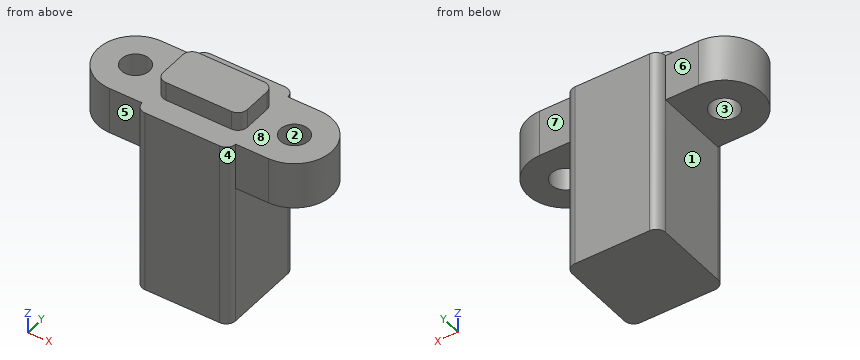
from build123d import *

# Parameters (mm, degrees)
SKETCH2_R           = 1.5
BOSS_EXTRUDE1_DEPTH = 5
BOSS_EXTRUDE2_DEPTH = 2
BOSS_EXTRUDE3_START = -15
SKETCH2_3_W         = 10
SKETCH2_3_H         = 4
BOSS_EXTRUDE3_DEPTH = 15


with BuildPart() as part:
    # Sketch2 → Boss-Extrude1 (new body)
    # profile 1 of 2: a face of its own
    with BuildSketch(Plane.XY):
        with BuildLine():
            Line((0, -4), (-17, -4))
            ThreePointArc((-17, -4), (-21, 0), (-17, 4))
            Line((-17, 4), (0, 4))
            ThreePointArc((0, 4), (4, 0), (0, -4))
        make_face()
        with Locations((-17, 0)):
            Circle(SKETCH2_R, mode=Mode.SUBTRACT)
        Circle(SKETCH2_R, mode=Mode.SUBTRACT)
    # profile 2 of 2: a face of its own
    with BuildSketch(Plane.XY):
        with BuildLine():
            Line((-12.5, 5), (-4.5, 5))
            ThreePointArc((-4.5, 5), (-3.792893219, 4.707106781), (-3.5, 4))
            Line((-3.5, 4), (-3.5, -4))
            ThreePointArc((-3.5, -4), (-3.792893219, -4.707106781), (-4.5, -5))
            Line((-4.5, -5), (-12.5, -5))
            ThreePointArc((-12.5, -5), (-13.207106781, -4.707106781), (-13.5, -4))
            Line((-13.5, -4), (-13.5, 4))
            ThreePointArc((-13.5, 4), (-13.207106781, 4.707106781), (-12.5, 5))
        make_face()
    extrude(amount=BOSS_EXTRUDE1_DEPTH)

    # Sketch3 → Boss-Extrude2 (add)
    with BuildSketch(Plane.XY.offset(5)):
        with BuildLine():
            Line((-12, -2.5), (-5, -2.5))
            ThreePointArc((-5, -2.5), (-4.292893219, -2.207106781), (-4, -1.5))
            Line((-4, -1.5), (-4, 1.5))
            ThreePointArc((-4, 1.5), (-4.292893219, 2.207106781), (-5, 2.5))
            Line((-5, 2.5), (-12, 2.5))
            ThreePointArc((-12, 2.5), (-12.707106781, 2.207106781), (-13, 1.5))
            Line((-13, 1.5), (-13, -1.5))
            ThreePointArc((-13, -1.5), (-12.707106781, -2.207106781), (-12, -2.5))
        make_face()
    extrude(amount=BOSS_EXTRUDE2_DEPTH)

    # Sketch2_3 → Boss-Extrude3 (add)
    with BuildSketch(Plane.XY.offset(BOSS_EXTRUDE3_START)):
        with BuildLine():
            Line((-13.5, 4), (-3.5, 4))
            ThreePointArc((-3.5, 4), (-3.792893219, 4.707106781), (-4.5, 5))
            Line((-4.5, 5), (-12.5, 5))
            ThreePointArc((-12.5, 5), (-13.207106781, 4.707106781), (-13.5, 4))
        make_face()
        with Locations((-8.5, 2)):
            Rectangle(SKETCH2_3_W, SKETCH2_3_H)
        with Locations((-8.5, -2)):
            Rectangle(SKETCH2_3_W, SKETCH2_3_H)
        with BuildLine():
            ThreePointArc((-4.5, -5), (-3.792893219, -4.707106781), (-3.5, -4))
            Line((-3.5, -4), (-13.5, -4))
            ThreePointArc((-13.5, -4), (-13.207106781, -4.707106781), (-12.5, -5))
            Line((-12.5, -5), (-4.5, -5))
        make_face()
    extrude(amount=BOSS_EXTRUDE3_DEPTH)


solid = part.part
Design review of the part built by this model. Coordinates are the model's own, in mm. Face numbers are marked on the shaded views. A direction names the side the tool comes from. Round coordinates to 2 decimals unless told otherwise and drop trailing zeros. Loops run counter-clockwise (first coordinate to the right, second up) from the corner with the lowest first, then second, coordinate; pieces in that order, holes last. Notation, with made-up numbers: (16.25, -16.5) - (66.25, -16.5) arc R31 cw to (66.25, 9.5) - close; hole circle Ø3 at (70.25, 5). An arc over 180 degrees is marked (long way). One line per question, with ' | ' between items.
1. We need section D-D, the plane z = -11. State the section outline as (x, y) points, and give its area (3 significant figures).
Results are:
outline: (-13.5, -4) arc R1 ccw to (-12.5, -5) - (-4.5, -5) arc R1 ccw to (-3.5, -4) - (-3.5, 4) arc R1 ccw to (-4.5, 5) - (-12.5, 5) arc R1 ccw to (-13.5, 4) - close | area: 99.1 mm²
2. For the marked faces 5, 6, 7 and 8, list the 3-axis set-ups (+Z, -Z, +X, -X, +Y, -Y) from which the entire face can be reached by the end or side of a thin tool; tool diameter is ignored.
Results are:
face 5: +Z, -Z, -X, -Y | face 6: +Z, -Z, -X, +Y | face 7: +Z, -Z, +X, +Y | face 8: +Z
3. Clearance check with flat-ended pins moving along their axes: P1, Ø1.6, axis at x = -9, z = 6.5, coming from the -Y side; P2, Ø4, axis at y = 2, z = -8, coming from the -X side; P3, Ø4, axis at y = 1, z = -10, coming from the +X side; P4, Ø6, axis at y = -1, z = 3.5, coming from the +X side. State where each tip first meets the part, or that it passes through.
Results are:
P1: stops at y = -2.5 | P2: stops at x = -13.5 | P3: stops at x = -3.5 | P4: stops at x = 4
4. Draft analysis for pull direction Y (two halves, no side actions). For the marked faces 1, 2, 3 and 4, state which applies: released by +Y, released by -Y, zero draft, split by the parting line, or undercut.
Results are:
face 1: zero draft | face 2: undercut | face 3: undercut | face 4: released by -Y
5. For L1, parallel to Y at x = -17, z = 2.9; L2, parallel to X at y = 1.25, z = 3; L3, parallel to Z at x = -5, y = 4, list the stretches that pass through material, from the lowest coordinate up. Write a range as [from, to].
Results are:
L1: y = [-4, -1.5], [1.5, 4] | L2: x = [-20.8, -17.83], [-16.17, -0.83], [0.83, 3.8] | L3: z = [-15, 5]
6. We need section C-C, the plane z = 3.5. State the section outline as (x, y) points, and give its area (3 significant figures).
Results are:
outline: (-17, -4) - (-13.5, -4) arc R1 ccw to (-12.5, -5) - (-4.5, -5) arc R1 ccw to (-3.5, -4) - (0, -4) arc R4 ccw to (0, 4) - (-3.5, 4) arc R1 ccw to (-4.5, 5) - (-12.5, 5) arc R1 ccw to (-13.5, 4) - (-17, 4) arc R4 ccw to start; hole circle Ø3 at (-17, 0); hole circle Ø3 at (0, 0) | area: 191 mm²
7. We need section A-A, the plane y = 0. State the section outline as (x, z) points, and give its area (3 significant figures).
Results are:
outline: (-21, 0) - (-18.5, 0) - (-18.5, 5) - (-21, 5) - close; (-15.5, 0) - (-13.5, 0) - (-13.5, -15) - (-3.5, -15) - (-3.5, 0) - (-1.5, 0) - (-1.5, 5) - (-4, 5) - (-4, 7) - (-13, 7) - (-13, 5) - (-15.5, 5) - close; (1.5, 0) - (4, 0) - (4, 5) - (1.5, 5) - close | area: 263 mm²
8. We need section B-B, the plane x = -7. State the section outline as (y, z) points, and give its area (3 significant figures).
Results are:
outline: (-5, -15) - (5, -15) - (5, 5) - (2.5, 5) - (2.5, 7) - (-2.5, 7) - (-2.5, 5) - (-5, 5) - close | area: 210 mm²
